from build123d import *
from build123d import SkipClean  # not in build123d's __all__

# Parameters (mm, degrees)
F0_R     = 5
F1_DEPTH = 20


with BuildPart() as f1:
    # F0 (on Front) → F1 (new body)
    with BuildSketch(Plane.XZ):
        with BuildLine():
            ThreePointArc((-15, 40), (-10.6066017178, 50.6066017178), (0, 55))
            Line((0, 55), (0, 60))
            ThreePointArc((0, 60), (-5, 65), (0, 70))
            Line((0, 70), (0, 75))
            ThreePointArc((0, 75), (-24.7487373415, 64.7487373415), (-35, 40))
            Line((-35, 40), (-35, 0))
            Line((-35, 0), (-30, 0))
            ThreePointArc((-30, 0), (-25, 5), (-20, 0))
            Line((-20, 0), (-15, 0))
            Line((-15, 0), (-15, 40))
        make_face()
        with Locations((-25, 20)):
            Circle(F0_R, mode=Mode.SUBTRACT)
        with Locations((-25, 40)):
            Circle(F0_R, mode=Mode.SUBTRACT)
        with Locations((-17.6776695297, 57.6776695297)):
            Circle(F0_R, mode=Mode.SUBTRACT)
    extrude(amount=F1_DEPTH)

    # F2: F1 across plane


with BuildPart() as f1_1:
    add(f1.part, clean=False)
    with SkipClean():  # cleaning this boolean's faces spoils the solid; the shape is the same uncleaned
        add(f1.part.mirror(Plane.YZ), clean=False)

    # F3: F1 across plane


with BuildPart() as f1_2:
    add(f1_1.part, clean=False)
    add(f1_1.part.mirror(Plane.XY), clean=False)


solid = f1_2.part
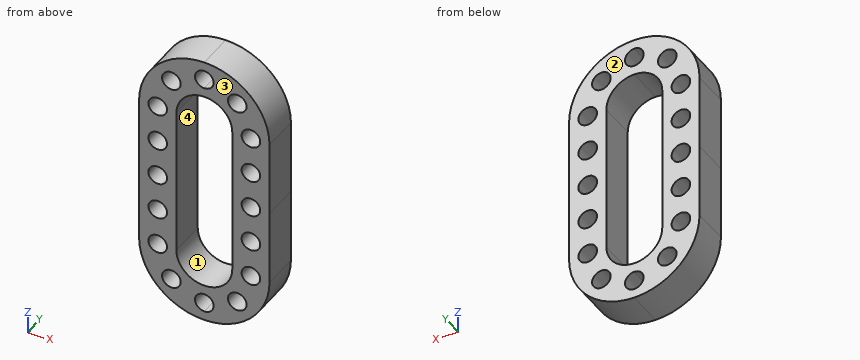
For this review, take the finished solid that the model builds, in its own axes (mm). Face numbers are marked on the shaded views. A direction names the side the tool comes from. Give positions to 0.01 mm unless a question says otherwise; leave off trailing zeros. Order: outer loops, then holes, each group sorted by start corner. A loop starts at its lowest first (then second) coordinate and runs counter-clockwise, first axis right, second up. Notation, with made-up numbers: M 52.5,-21.5 L 79.5,-21.5 A9 cw 79.5,-5.5 Z; hole C -19,81.5 d7. An arc over 180 degrees is marked long. Answer in a Markdown table with one row per item. Add a question column.
(1) Consider section D-D on y = -7.5. Give the number of separate pieces and of enclosed holes in the cut face, and give its area (3 significant figures).
(2) Wall thickness on probe 1 along Z at (x, y) = (18, -15); probe 2 along X at (y, z) = (-10, -20); probe 3 along Z at (x, y) = (23, -14.5): over which ranges is each line inside the solid? List them lowest first. Write a range as [from, to].
(3) Mouldability with a two-part tool opening along X and no side actions: class the marked faces 1 and 2 as +X half, -X half, draft (parallel to the pull), parting line (faces both ways), or undercut.
(4) Consider section A-A on x = -28. State the section outline as (y, z) points.
(5) Consider section C-C on z = -20. State the section outline as (x, y) points, and give its area (3 significant figures).
(6) Consider section B-B on z = 26.5. State the section outline as (x, y) points.
(7) For the marked faces 3 and 4, list the 3-axis set-ups (+Z, -Z, +X, -X, +Y, -Y) from which the entire face can be reached by the end or side of a thin tool; tool diameter is ignored.
(8) For pin 1 (8 mm diameter, centred on x = 17.68, z = 57.68, fed in from -Y); pin 2 (1.5 mm diameter, centred on x = 24.5, y = -18, fed in from +Z); pin 3 (1 mm diameter, centred on y = -10, z = -50, fed in from -X); pin 4 (2 mm diameter, centred on x = 16, y = -9, fed in from -Z), all flat-tipped, find the tip position at first contact; note any pin that passes through.
Evaluation:
| question | item | result |
|---|---|---|
| 1 | separate pieces | 1 |
| 1 | enclosed holes | 17 |
| 1 | area | 5,080 mm^2 |
| 2 | probe 1 | z = [-70.02, -62.67], [-52.69, 52.69], [62.67, 70.02] |
| 2 | probe 2 | x = [-35, -30], [-20, -15], [15, 20], [30, 35] |
| 2 | probe 3 | z = [-66.38, -44.58], [-35.42, -24.58], [-15.42, -4.58], [4.58, 15.42], [24.58, 35.42], [44.58, 66.38] |
| 3 | face 1 | undercut |
| 3 | face 2 | draft |
| 4 | outline | M -20,-61 L 0,-61 L 0,-44 L -20,-44 Z; M -20,-36 L 0,-36 L 0,-24 L -20,-24 Z; M -20,-16 L 0,-16 L 0,-4 L -20,-4 Z; M -20,4 L 0,4 L 0,16 L -20,16 Z; M -20,24 L 0,24 L 0,36 L -20,36 Z; M -20,44 L 0,44 L 0,61 L -20,61 Z |
| 5 | outline | M -35,-20 L -30,-20 L -30,0 L -35,0 Z; M -20,-20 L -15,-20 L -15,0 L -20,0 Z; M 15,-20 L 20,-20 L 20,0 L 15,0 Z; M 30,-20 L 35,-20 L 35,0 L 30,0 Z |
| 5 | area | 400 mm^2 |
| 6 | outline | M -35,-20 L -15,-20 L -15,0 L -35,0 Z; M 15,-20 L 35,-20 L 35,0 L 15,0 Z |
| 7 | face 3 | +Z, -Z, +X, -X, -Y |
| 7 | face 4 | +Y, -Y |
| 8 | pin 1 | passes through |
| 8 | pin 2 | stops at z = 65.71 |
| 8 | pin 3 | stops at x = -33.69 |
| 8 | pin 4 | stops at z = -71.62 |
